Geometry check sheet. Reference: the model listing, model coordinates, mm. Face numbers are marked on the shaded views. A direction names the side the tool comes from. Give positions to 0.01 mm unless a question says otherwise; leave off trailing zeros. Write each loop counter-clockwise with the first axis right and the second up, starting at its lowest first coordinate (ties: lowest second). Pieces come first, ordered by that corner, then holes. Notation, with made-up numbers: M -9.75,66 L -1.75,66 A23 ccw -1.75,91 Z; hole C 69,53 d9. An arc over 180 degrees is marked long. One line per item, written item: value. Start each with the question number.
1. Cross-section at B-B on y = 4. Record the cut outline in (x, z).
2. Tool access check on the marked faces 4, 5 and 6. Record the directions out of +Z, -Z, +X, -X, +Y, -Y that give a thin tool (end or side, any length) a straight path to the whole face; none if there is none.
3. Gauge pin test, flat ends, axial feed: pin 1 (8 mm diameter, centred on x = 38.5, y = 1, fed in from -Z); pin 2 (6 mm diameter, centred on x = 38, z = -9, fed in from +Y) (3 decimals); pin 3 (2 mm diameter, centred on x = 17, z = -1.5, fed in from +Y). Record the tip position at first contact, or that the pin passes through.
4. Cross-section at D-D on y = 7.75. Record the cut outline in (x, z).
5. Scan lines: line 1 (Y direction, x = 0, z = -1.5); line 2 (Z direction, x = 11.5, y = -7.5); line 3 (Z direction, x = 0, y = 7). Record each from-to range of solid material in increasing order.
6. Cross-section at C-C on z = -4.25. Record the cut outline in (x, y), then the cut area to 3 significant figures.
7. Cross-section at A-A on x = 0. Record the cut outline in (y, z).
8. Release check for a two-part mould opening along X. For the marked faces 1, 2 and 3 record: pulls with the +X half, pulls with the -X half, needs draft (parallel to the pull), parting line crosses it, or undercut.
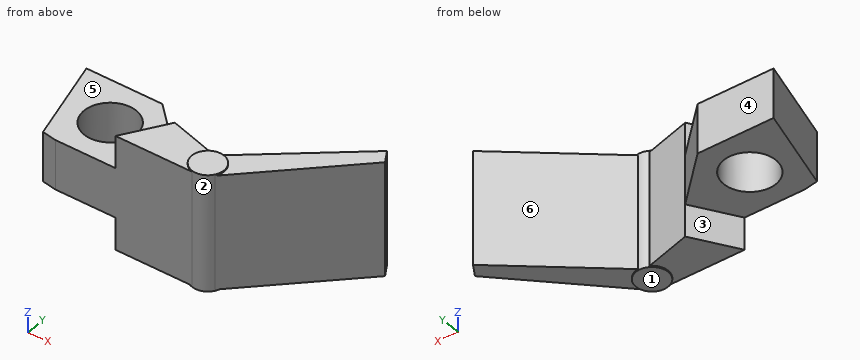
from build123d import *

# Parameters (mm, degrees)
SKETCH2_R           = 9
SKETCH2_R_2         = 5.25
BOSS_EXTRUDE1_DEPTH = 5
BOSS_EXTRUDE2_DEPTH = 11.5
SKETCH2_16_R        = 3.25
BOSS_EXTRUDE3_DEPTH = 11.75
CUT_EXTRUDE1_DEPTH  = 10
BOSS_EXTRUDE4_DEPTH = 10


with BuildPart() as part:
    # Sketch2 → Boss-Extrude1 (new, symmetric)
    # profile 1 of 4: a face of its own
    with BuildSketch(Plane.XY):
        Circle(SKETCH2_R)
        Circle(SKETCH2_R_2, mode=Mode.SUBTRACT)
    # profile 2 of 4: a face of its own
    with BuildSketch(Plane.XY):
        with BuildLine():
            Line((-9, 9), (-9, 0))
            ThreePointArc((-9, 0), (-6.363961031, 6.363961031), (0, 9))
            Line((0, 9), (-9, 9))
        make_face()
    # profile 3 of 4: a face of its own
    with BuildSketch(Plane.XY):
        with BuildLine():
            Line((-9, -9), (0, -9))
            ThreePointArc((0, -9), (-6.363961031, -6.363961031), (-9, 0))
            Line((-9, 0), (-9, -9))
        make_face()
    # profile 4 of 4: a face of its own
    with BuildSketch(Plane.XY):
        with BuildLine():
            ThreePointArc((9, 0), (6.363961031, -6.363961031), (0, -9))
            Line((0, -9), (8, -9))
            Line((8, -9), (13.404247693, -0.419567503))
            Line((13.404247693, -0.419567503), (3.65, 9))
            Line((3.65, 9), (0, 9))
            ThreePointArc((0, 9), (6.363961031, 6.363961031), (9, 0))
        make_face()
    extrude(amount=BOSS_EXTRUDE1_DEPTH, both=True)

    # Sketch2_15 → Boss-Extrude2 (add, symmetric)
    with BuildSketch(Plane.XY):
        with BuildLine():
            Line((13.404247693, -0.419567503), (8, -9))
            Line((8, -9), (23.45, -9))
            ThreePointArc((23.45, -9), (21.073071329, -6.303811499), (22.634247693, -3.066227414))
            Line((22.634247693, -3.066227414), (13.404247693, -0.419567503))
        make_face()
        with BuildLine():
            ThreePointArc((27.542787913, -5.861177206), (27.416408735, -6.7586698), (27.047099939, -7.586362779))
            Line((27.047099939, -7.586362779), (46.492536422, 11.859073704))
            Line((46.492536422, 11.859073704), (44.932659612, 14.404893086))
            Line((44.932659612, 14.404893086), (24.632481869, -2.628978571))
            ThreePointArc((24.632481869, -2.628978571), (26.708000673, -3.686493937), (27.542787913, -5.861177206))
        make_face()
    extrude(amount=BOSS_EXTRUDE2_DEPTH, both=True)


with BuildPart() as boss_extrude2_piece_1:
    # of the separate pieces the step leaves, piece 1, a body of its own (boss_extrude2_pieces)
    add(part.part.solids().sort_by_distance((22.634247693, -3.066227414, -11.5))[0])



with BuildPart() as boss_extrude2_piece_2:
    # of the separate pieces the step leaves, piece 2, a body of its own (boss_extrude2_pieces)
    add(part.part.solids().sort_by_distance((24.632481869, -2.628978571, -11.5))[0])


with BuildPart() as boss_extrude2_piece_1_1:
    add(boss_extrude2_piece_1.part)

    add(boss_extrude2_piece_2.part)  # Boss-Extrude3 merges Boss-Extrude2 piece 2
    # Sketch2_16 → Boss-Extrude3 (add, symmetric)
    with BuildSketch(Plane.XY):
        with Locations((24.292787913, -5.861177206)):
            Circle(SKETCH2_16_R)
    extrude(amount=BOSS_EXTRUDE3_DEPTH, both=True)

    # Sketch3 → Cut-Extrude1 (cut)
    with BuildSketch(Plane(origin=(0, 0, -5), x_dir=(-1, 0, 0), z_dir=(0, 0, -1))):
        Polygon((9, 9), (9, -9), (4.176914536, -9), align=None)
    extrude(amount=-CUT_EXTRUDE1_DEPTH, mode=Mode.SUBTRACT)

    # Sketch4 → Boss-Extrude4 (add)
    with BuildSketch(Plane(origin=(0, 0, -5), x_dir=(-1, 0, 0), z_dir=(0, 0, -1))):
        Polygon((9, 9), (11.729028356, 9), (7.033855882, -8.522622223), (4.176914536, -9), align=None)
    extrude(amount=-BOSS_EXTRUDE4_DEPTH)


solid = boss_extrude2_piece_1_1.part
Report:
1. outline: M -10.39,-5 L -3.4,-5 L -3.4,5 L -10.39,5 Z; M 3.4,-5 L 8.83,-5 L 8.83,5 L 3.4,5 Z; M 32.53,-11.5 L 38.63,-11.5 L 38.63,11.5 L 32.53,11.5 Z
2. face 4: +Z, -Z, -X, +Y
2. face 5: +Z, -X, +Y
2. face 6: +Z, -Z, +Y
3. pin 1: stops at z = -11.5
3. pin 2: stops at y = 11.105
3. pin 3: stops at y = -1.16
4. outline: M -11.39,-5 L 4.94,-5 L 4.94,5 L -11.39,5 Z; M 37,-11.5 L 42.38,-11.5 L 42.38,11.5 L 37,11.5 Z
5. line 1: y = -9 to -5.25, 5.25 to 9
5. line 2: z = -11.5 to 11.5
5. line 3: z = -5 to 5
6. outline: M -11.73,9 L -7.03,-8.52 L -4.18,-9 L 23.45,-9 A3.25 ccw 27.05,-7.59 L 46.49,11.86 L 44.93,14.4 L 24.63,-2.63 A3.25 ccw 22.63,-3.07 L 13.4,-0.42 L 3.65,9 Z; hole C 0,0 d10.5
6. area: 475 mm^2
7. outline: M -9,-5 L -5.25,-5 L -5.25,5 L -9,5 Z; M 5.25,-5 L 9,-5 L 9,5 L 5.25,5 Z
8. face 1: needs draft
8. face 2: undercut
8. face 3: pulls with the -X half
